from build123d import *

# Parameters (mm, degrees)
SKETCH1_R           = 9.5
SKETCH1_R_2         = 7.5
BOSS_EXTRUDE1_DEPTH = 100
SKETCH2_W           = 5.2
SKETCH2_H           = 94
CUT_EXTRUDE1_DEPTH  = 100


with BuildPart() as part:
    # Sketch1 → Boss-Extrude1 (new body)
    with BuildSketch(Plane(origin=(0, 0, 0), x_dir=(1, 0, 0), z_dir=(0, 1, 0))):
        with Locations(Location((0, 0, 0), (0, 0, 270))):
            Circle(SKETCH1_R)
        with Locations(Location((0, 0, 0), (0, 0, 270))):
            Circle(SKETCH1_R_2, mode=Mode.SUBTRACT)
    extrude(amount=BOSS_EXTRUDE1_DEPTH)

    # Sketch2 → Cut-Extrude1 (cut)
    with BuildSketch(Plane.XY.offset(20)):
        with Locations((0, 47)):
            Rectangle(SKETCH2_W, SKETCH2_H)
    extrude(amount=-CUT_EXTRUDE1_DEPTH, mode=Mode.SUBTRACT)


solid = part.part
Work out the finished part from the listing and answer in its coordinate system (mm). A direction names the side the tool comes from. Give positions to 0.01 mm unless a question says otherwise; leave off trailing zeros. Loops run counter-clockwise (first coordinate to the right, second up) from the corner with the lowest first, then second, coordinate; pieces in that order, holes last. Notation, with made-up numbers: (1.25, 57.5) - (7.25, 57.5) arc R24 cw to (7.25, 78.5) - close; hole circle Ø7 at (36.25, -7). An arc over 180 degrees is marked (long way). Answer in a Markdown table with one row per item. Add a question column.
Q1. Consider line 1 along X through (y, z) = (40, 0); line 2 along X through (y, z) = (15.5, -4.25); line 3 along Z through (x, y) = (6.5, 88.5). Determine where each line is inside the solid, lowest interval first.
Q2. The part is cut by section B-B (z = 0). Determine the outline of the cut face in (x, y).
Q3. The part is cut by section A-A (y = 92.5). Determine the outline of the cut face in (x, z), and give its area (3 significant figures).
Q4. Determine the mould class of faces 3 (the cylindrical face through (2.854, 49.3, 9.061)), 4 (the flat face through (2.6, 46, -8)), 5 (the flat face through (-8, 0, 0)) for opening direction X: released by +X, released by -X, zero draft, split by the parting line, or undercut.
Q5. Each of these flat-tipped pins is pushed along its axis until it touches: P1, Ø1.1, axis at y = 30, z = 8.5, coming from the -X side; P2, Ø5, axis at x = -4.5, z = -5.5, coming from the -Y side; P3, Ø3, axis at x = 4, y = 15, coming from the -Z side; P4, Ø10, axis at x = 1, y = 29, coming from the +Z side. Where does it stop, or does it pass through?
Q6. A tool of negligible diameter and unlimited length cuts with its end or side. For faces 1 (the cylindrical face through (-7.32, 49.3, -1.63)), 2 (the flat face through (-2.6, 46, -8)), from which of +Z, -Z, +X, -X, +Y, -Y can it reach the whole face along a straight path? Write none if from no direction.
Solution:
| question | item | result |
|---|---|---|
| 1 | line 1 | x = -9.5 to -7.5, 7.5 to 9.5 |
| 1 | line 2 | x = -8.5 to -6.18, 6.18 to 8.5 |
| 1 | line 3 | z = -6.93 to -3.74, 3.74 to 6.93 |
| 2 | outline | (-9.5, 0) - (-7.5, 0) - (-7.5, 100) - (-9.5, 100) - close; (7.5, 0) - (9.5, 0) - (9.5, 100) - (7.5, 100) - close |
| 3 | outline | (-2.6, -9.14) - (-2.6, -7.03) arc R7.5 cw to (-2.6, 7.03) - (-2.6, 9.14) arc R9.5 ccw to start; (2.6, -9.14) arc R9.5 ccw to (2.6, 9.14) - (2.6, 7.03) arc R7.5 cw to (2.6, -7.03) - close |
| 3 | area | 85.7 mm² |
| 4 | face 3 | split by the parting line |
| 4 | face 4 | undercut |
| 4 | face 5 | zero draft |
| 5 | P1 | stops at x = -5.2 |
| 5 | P2 | stops at y = 0 |
| 5 | P3 | stops at z = -9.14 |
| 5 | P4 | stops at z = 9.14 |
| 6 | face 1 | +Y, -Y |
| 6 | face 2 | +Z, -Z, -Y |
